Design review of the part built by this model. Coordinates are the model's own, in mm. A direction names the side the tool comes from. Coordinates: 2 decimals unless noted, no trailing zeros. Loops run counter-clockwise (first coordinate to the right, second up) from the corner with the lowest first, then second, coordinate; pieces in that order, holes last. Notation, with made-up numbers: M 59.5,4.5 L 103.5,4.5 A7 ccw 103.5,10.5 Z; hole C 89,57.25 d2. An arc over 180 degrees is marked long. Put each result on its own line as item: value. Start each with the question number.
(1) Take a section at A-A, the plane z = -16. Give the boundary of the cut face in (x, y), then the cut area to 3 significant figures.
(2) For probe 1 along Y at (x, z) = (-0.2, 10.5); probe 2 along Y at (x, z) = (-12, 33.5); probe 3 along X at (y, z) = (2.75, 3), list the stretches that pass through material, from the lowest coordinate up. Write a range as [from, to].
(3) Take a section at B-B, the plane y = -9.25. Give the boundary of the cut face in (x, z).
(4) Take a section at C-C, the plane z = 10.5. Give the boundary of the cut face in (x, y).
(5) The part is to be moulded in two halves that separate along Z. For faces 1 (the flat face through (0, 6, 22.5)), 2 (the cylindrical face through (0, 0, -12)), 3 (the flat face through (0, -12.5, 0)), say which applies: +Z half, -Z half, draft (parallel to the pull), parting line (faces both ways), or undercut.
(6) Clearance check with flat-ended pins moving along their axes: pin 1 (5 mm diameter, centred on x = -2, y = -1.5, fed in from +Z); pin 2 (7 mm diameter, centred on x = -3.5, z = 27, fed in from +Y); pin 3 (1.6 mm diameter, centred on x = -0.5, y = 8, fed in from +Z). State where each tip first meets the part, or that it passes through.
(7) For faces 4 (the flat face through (-6.7, 0, 29.5)), 5 (the flat face through (-1, 0, 0)), 6 (the flat face through (-6.7, -6, 29.5)), list the 3-axis set-ups (+Z, -Z, +X, -X, +Y, -Y) from which the entire face can be reached by the end or side of a thin tool; tool diameter is ignored.
(8) Take a section at D-D, the plane x = -3.25. Give the boundary of the cut face in (y, z), then the cut area to 3 significant figures.
```python
from build123d import *

# Parameters (mm, degrees)
SKETCH1_W           = 2
SKETCH1_H           = 45
BOSS_EXTRUDE1_DEPTH = 12.5
BOSS_EXTRUDE2_START = -12.5
BOSS_EXTRUDE2_DEPTH = 6
SKETCH3_R           = 2.5
CUT_EXTRUDE1_DEPTH  = 3


with BuildPart() as part:
    # Sketch1 → Boss-Extrude1 (new, symmetric)
    with BuildSketch(Plane(origin=(0, 0, 0), x_dir=(1, 0, 0), z_dir=(0, 1, 0))):
        Rectangle(SKETCH1_W, SKETCH1_H)
    extrude(amount=BOSS_EXTRUDE1_DEPTH, both=True)

    # Sketch2 → Boss-Extrude2 (add)
    with BuildSketch(Plane(origin=(0, 12.5, 0), x_dir=(1, 0, 0), z_dir=(0, 1, 0)).offset(BOSS_EXTRUDE2_START)):
        with BuildLine():
            Line((1, -22.5), (1, -22.509542629))
            ThreePointArc((1, -22.509542629), (0.827090915, -23.323015916), (0.338261213, -23.99583228))
            Line((0.338261213, -23.99583228), (-13.417009614, -36.381133763))
            ThreePointArc((-13.417009614, -36.381133763), (-13.849889552, -36.534424589), (-14.264374873, -36.336725232))
            Line((-14.264374873, -36.336725232), (-14.356889682, -36.233977127))
            ThreePointArc((-14.356889682, -36.233977127), (-14.510180508, -35.80109719), (-14.312481151, -35.386611868))
            Line((-14.312481151, -35.386611868), (-1.661738787, -23.99583228))
            ThreePointArc((-1.661738787, -23.99583228), (-1.172909085, -23.323015916), (-1, -22.509542629))
            Line((-1, -22.509542629), (-1, -22.5))
            Line((-1, -22.5), (1, -22.5))
        make_face()
    extrude(amount=-BOSS_EXTRUDE2_DEPTH)

    # Sketch3 → Cut-Extrude1 (cut, symmetric)
    with BuildSketch(Plane(origin=(1, 0, 0), x_dir=(0, 0, -1), z_dir=(1, 0, 0))):
        with Locations((-10.5, 0)):
            Circle(SKETCH3_R)
        with Locations((14.5, 0)):
            Circle(SKETCH3_R)
    extrude(amount=CUT_EXTRUDE1_DEPTH, both=True, mode=Mode.SUBTRACT)


solid = part.part
```
Computed values:
1. outline: M -1,-12.5 L 1,-12.5 L 1,-2 L -1,-2 Z; M -1,2 L 1,2 L 1,12.5 L -1,12.5 Z
1. area: 42.0 mm^2
2. probe 1: y = [-12.5, -2.5], [2.5, 12.5]
2. probe 2: y = [-6, 0]
2. probe 3: x = [-1, 1]
3. outline: M -1,-22.5 L 1,-22.5 L 1,22.5 L -1,22.5 Z
4. outline: M -1,-12.5 L 1,-12.5 L 1,-2.5 L -1,-2.5 Z; M -1,2.5 L 1,2.5 L 1,12.5 L -1,12.5 Z
5. face 1: +Z half
5. face 2: undercut
5. face 3: draft
6. pin 1: stops at z = 28.35
6. pin 2: stops at y = 0
6. pin 3: stops at z = 22.5
7. face 4: +Z, +X, -X, +Y
7. face 5: -Z, -X, +Y, -Y
7. face 6: +Z, +X, -X, -Y
8. outline: M -6,25.43 L 0,25.43 L 0,27.23 L -6,27.23 Z
8. area: 10.8 mm^2
